Study the drawing (mm; zero at the part's minimum x, y, z) and answer. A direction names the side the tool comes from. Round coordinates to 2 decimals unless told otherwise and drop trailing zeros. Loops run counter-clockwise (first coordinate to the right, second up) from the corner with the lowest first, then second, coordinate; pieces in that order, holes last. Notation, with made-up numbers: (64, 73) - (96, 73) arc R26 ccw to (96, 99) - close; hole circle Ø6 at (-14.75, -8.75). An arc over 180 degrees is marked (long way). Use CSV: the item, a comma, the result in double quotes. Start each with the question number.
1. A tool of negligible diameter and unlimited length cuts with its end or side. For the marked faces 4 and 5, from which of +Z, -Z, +X, -X, +Y, -Y can it reach the whole face along a straight path? Write none if from no direction.
2. Find section D-D (x = 56.5). Give the vertices of the cut face in (y, z), and give its area (3 significant figures).
3. Find section A-A (y = 12.5). Give the vertices of the cut face in (x, z).
4. Given pin 1 Ø8 at (x, z) = (27, 11) entering from -Y; pin 2 Ø5 at (x, y) = (60.5, 11) entering from -Z; pin 3 Ø6 at (x, z) = (16, 4.5) entering from -Y, each flat-ended and moving along its own axis, determine where each tip first touches the part or whether it passes through.
5. Find section C-C (z = 15). Give the vertices of the cut face in (x, y), and give its area (3 significant figures).
6. Consider line 1 along X through (y, z) = (2, 16.75); line 2 along Y through (x, z) = (26, 13); line 3 along Z through (x, y) = (52, 14.5). Determine where each line is inside the solid, lowest interval first.
7. Determine the mould class of the marked faces 1, 2 and 3 for opening direction X: +X half, -X half, draft (parallel to the pull), parting line (faces both ways), or undercut.
8. Find section B-B (z = 21). Give the vertices of the cut face in (x, y).
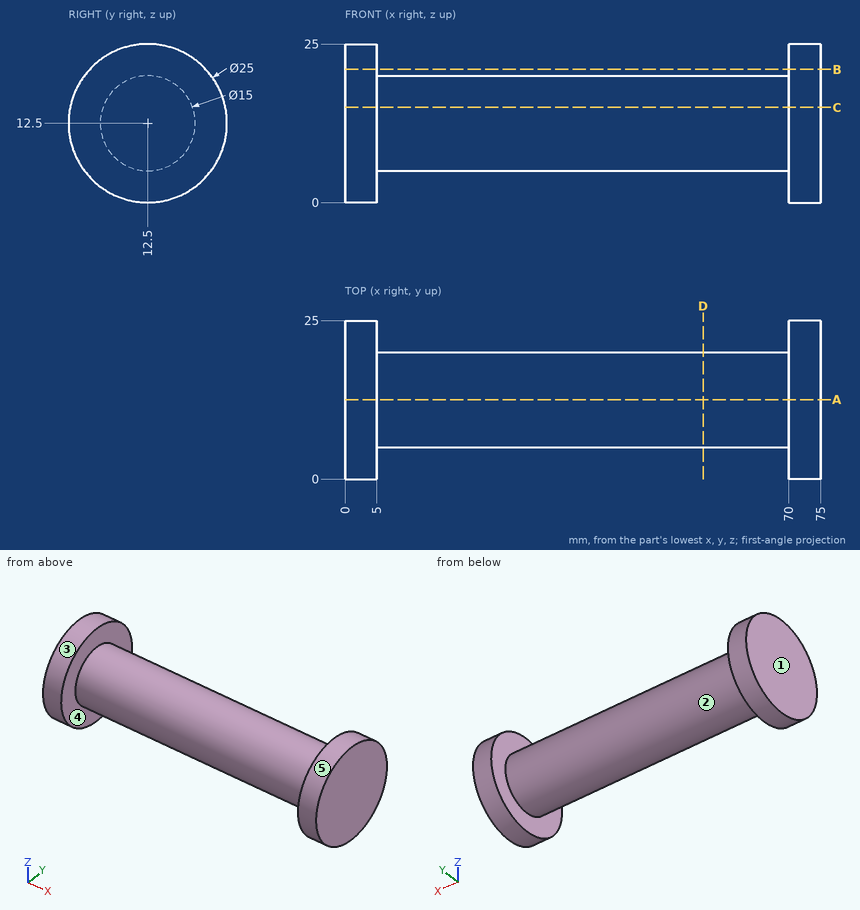
Filled sheet:
1,face 4,"none"
1,face 5,"+X, -X"
2,outline,"circle Ø15 at (12.5, 12.5)"
2,area,"177 mm²"
3,outline,"(0, 0) - (5, 0) - (5, 5) - (70, 5) - (70, 0) - (75, 0) - (75, 25) - (70, 25) - (70, 20) - (5, 20) - (5, 25) - (0, 25) - close"
4,pin 1,"stops at y = 5"
4,pin 2,"stops at z = 5"
4,pin 3,"stops at y = 6.91"
5,outline,"(0, 0.25) - (5, 0.25) - (5, 5.43) - (70, 5.43) - (70, 0.25) - (75, 0.25) - (75, 24.75) - (70, 24.75) - (70, 19.57) - (5, 19.57) - (5, 24.75) - (0, 24.75) - close"
5,area,"1,160 mm²"
6,line 1,"x = 0 to 5, 70 to 75"
6,line 2,"y = 5.02 to 19.98"
6,line 3,"z = 5.27 to 19.73"
7,face 1,"-X half"
7,face 2,"undercut"
7,face 3,"draft"
8,outline,"(0, 3.33) - (5, 3.33) - (5, 21.67) - (0, 21.67) - close; (70, 3.33) - (75, 3.33) - (75, 21.67) - (70, 21.67) - close"
